CAD build for the part. Positions are in the model's coordinates, mm. Face numbers are marked on the shaded views. A direction names the side the tool comes from. Give positions to 0.01 mm unless a question says otherwise; leave off trailing zeros. Loops run counter-clockwise (first coordinate to the right, second up) from the corner with the lowest first, then second, coordinate; pieces in that order, holes last. Notation, with made-up numbers: (7.5, 55.25) - (27.5, 55.25) arc R16 ccw to (27.5, 64.25) - close; hole circle Ø8 at (85, 86.5). An arc over 180 degrees is marked (long way). Return JSON: item names as keys, results as strings.
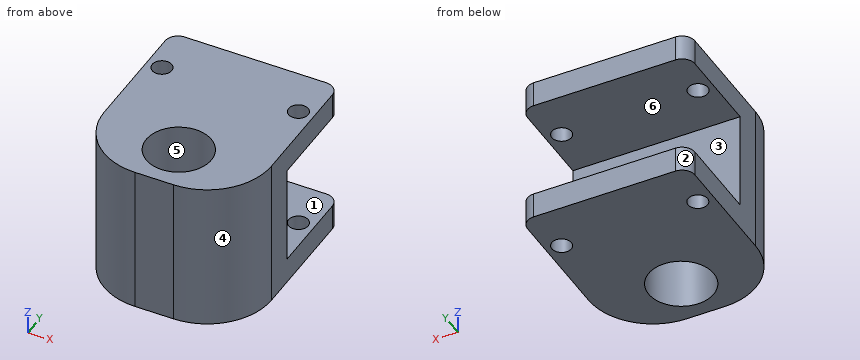
Autodesk Inventor part; units mm, degrees
ref_plane "YZ Plane" through (0, 0, 0) normal (1, 0, 0) x (0, 1, 0)
ref_plane "XZ Plane" through (0, 0, 0) normal (0, 1, 0) x (-1, 0, 0)
ref_plane "XY Plane" through (0, 0, 0) normal (0, 0, 1) x (1, 0, 0)
ref_plane "Work Plane1" through (0, 0, 0) normal (0, 0, 1) x (1, 0, 0)
sketch "Sketch1" plane through (0, 0, 0) normal (0, 0, 1) x (1, 0, 0)
  line L0 (-9.7566, -4.627) -> (-9.7566, 4.627) construction
  line L1 (-9.7566, -9.525) -> (-314.5566, -9.525) construction
  line L2 (-9.7566, 9.525) -> (-314.5566, 9.525) construction
  line L3 (-42.7766, 3) -> (-42.7766, -3) construction
  line L4 (-9.7566, 9.525) -> (-42.7766, 9.525)
  line L5 (-42.7766, 9.525) -> (-42.7766, -9.525)
  line L6 (-9.7566, -9.525) -> (-9.7566, 9.525)
  line L7 (-9.7566, -9.525) -> (-9.7566, -28.575)
  line L8 (-9.7566, -28.575) -> (-42.7766, -28.575)
  line L9 (-42.7766, -28.575) -> (-42.7766, -9.525)
  arc A0 (-38.0982, 0.6213) -> (-38.1469, -0.737) centre (-39.737, 0) ccw construction
  arc A1 (-11.1575, 0.6213) -> (-11.2061, -0.737) centre (-12.7962, 0) ccw construction
  circle A2 centre (-12.7962, 0) radius 1.9304
  circle A3 centre (-39.737, 0) radius 1.9304
  point P0 (0, 0)
  dimension "d1" = 19.05
  dimension "d2" = 3.8608
  dimension "d3" = 3.8608
extrude "Extrusion1" add sketch "Sketch1" along normal blind 5.08
ref_plane "Work Plane2" through (0, 0, -19.558) normal (0, 0, -1) x (-1, 0, 0)
sketch "Sketch2" plane through (0, 0, -19.558) normal (0, 0, -1) x (-1, 0, 0)
  line L0 (9.7566, -28.575) -> (9.7566, 9.525)
  line L1 (42.7766, 9.525) -> (42.7766, -28.575)
  line L2 (9.7566, 9.525) -> (42.7766, 9.525)
  line L3 (42.7766, 9.525) -> (42.7766, -28.575)
  line L4 (42.7766, -28.575) -> (9.7566, -28.575)
  line L5 (9.7566, -28.575) -> (9.7566, 9.525)
  circle A0 centre (12.7962, 0) radius 1.9304
  circle A1 centre (12.7962, 0) radius 1.9304
  circle A2 centre (39.6875, 0) radius 1.9304
  point P0 (0, 0)
  dimension "d7" = 3.8608
  dimension "d8" = 3.8608
  dimension "d24" = 38.1
  dimension "d25" = 9.525
  dimension "d26" = 26.8913
extrude "Extrusion2" add sketch "Sketch2" along normal blind 5.08
sketch "Sketch3" plane through (0, 0, 0) normal (0, 0, -1) x (-1, 0, 0)
  line L0 (9.7566, 9.525) -> (42.7766, 9.525) construction
  line L1 (9.7566, 9.525) -> (42.7766, 9.525) construction
  line L2 (42.7766, 9.525) -> (42.7766, -9.525) construction
  line L3 (42.7766, -9.525) -> (9.7566, -9.525) construction
  line L4 (9.7566, -9.525) -> (9.7566, 9.525) construction
  line L5 (42.7766, -28.575) -> (9.7566, -28.575)
  line L6 (42.7766, -10.033) -> (42.7766, -28.575)
  line L7 (42.7766, -28.575) -> (9.7566, -28.575)
  line L8 (9.7566, -28.575) -> (9.7566, -10.033)
  line L9 (42.7766, 9.525) -> (42.7766, -28.575)
  line L10 (42.7766, -10.033) -> (9.7566, -10.033)
  point P0 (0, 0)
  dimension "d11" = 19.05
extrude "Extrusion3" add sketch "Sketch3" along normal up to surface (19.558 mm away)
sketch "Sketch4" plane through (0, 0, -24.638) normal (0, 0, -1) x (-1, 0, 0)
  circle A0 centre (26.2666, -19.304) radius 6.4135
  line L0 (9.7566, -28.575) -> (42.7766, -28.575)
  line L1 (42.7766, -28.575) -> (42.7766, 9.525)
  line L2 (9.7566, 9.525) -> (9.7566, -28.575)
  line L3 (42.7766, -10.033) -> (9.7566, -10.033) construction
  point P0 (0, 0)
  dimension "d15" = 12.827
  dimension "d16" = 9.271
  dimension "d17" = 33.02
  dimension "d18" = 16.51
  dimension "d19" = 18.542
extrude "Extrusion4" cut sketch "Sketch4" against normal through all
fillet "Fillet1" radius 12.7 2 edges at (-9.7566, -28.575, -9.779) (-42.7766, -28.575, -9.779)
fillet "Fillet2" radius 2.54 4 edges at (-9.7566, 9.525, -22.098) (-9.7566, 9.525, 2.54) (-42.7766, 9.525, -22.098) (-42.7766, 9.525, 2.54)
equation "\"d16\" = 0.5 * d19"
equation "\"d18\" = 0.5 * d17"
properties part number "Bearing mount for xrail"
1. Pull direction Y, two halves, no side cores. Call the marked faces 3, 4, 5 and 6: +Y half, -Y half, draft (parallel to the pull), parting line (faces both ways), or undercut.
Values follow:
{"face 3": "+Y half", "face 4": "-Y half", "face 5": "undercut", "face 6": "draft"}
2. Cut at C-C, the plane z = -2.25. Write the cut outline in (x, y) (1 decimal), plus the area to 3 significant figures.
Values follow:
{"outline": "(-42.8, -15.9) arc R12.7 ccw to (-30.1, -28.6) - (-22.5, -28.6) arc R12.7 ccw to (-9.8, -15.9) - (-9.8, -10) - (-42.8, -10) - close; hole circle Ø12.8 at (-26.3, -19.3)", "area": "414 mm²"}
3. Which spindle directions (+Z, -Z, +X, -X, +Y, -Y) get a long thin tool onto all of the face, cutting with end or side? Do the marked faces 1 and 2. Say none if no direction does.
Values follow:
{"face 1": "+X, -X, +Y", "face 2": "+Z, -Z, -X, +Y"}
4. Drill centre lines: probe 1 along Z at (x, y) = (-26.5, -10); probe 2 along Y at (x, z) = (-30.5, -7.75); probe 3 along Y at (x, z) = (-28.5, -3.25) (3 decimals). Where is each one in solid material? Low to high.
Values follow:
{"probe 1": "z = -24.64 to -19.56, 0 to 5.08", "probe 2": "y = -28.57 to -24.12, -14.49 to -10.03", "probe 3": "y = -28.575 to -25.316, -13.292 to -10.033"}
5. Cut at D-D, the plane y = -21. Write the cut outline in (x, z), plus the area to 3 significant figures.
Values follow:
{"outline": "(-41.7, -24.64) - (-32.45, -24.64) - (-32.45, 5.08) - (-41.7, 5.08) - close; (-20.08, -24.64) - (-10.84, -24.64) - (-10.84, 5.08) - (-20.08, 5.08) - close", "area": "549 mm²"}
6. Cut at A-A, the plane y = 0. Write the cut outline in (x, z).
Values follow:
{"outline": "(-42.78, -24.64) - (-41.62, -24.64) - (-41.62, -19.56) - (-42.78, -19.56) - close; (-42.78, 0) - (-41.67, 0) - (-41.67, 5.08) - (-42.78, 5.08) - close; (-37.81, 0) - (-14.73, 0) - (-14.73, 5.08) - (-37.81, 5.08) - close; (-37.76, -24.64) - (-14.73, -24.64) - (-14.73, -19.56) - (-37.76, -19.56) - close; (-10.87, -24.64) - (-9.76, -24.64) - (-9.76, -19.56) - (-10.87, -19.56) - close; (-10.87, 0) - (-9.76, 0) - (-9.76, 5.08) - (-10.87, 5.08) - close"}
7. Cut at B-B, the plane x = -14. Write the cut outline in (y, z) (3 decimals), plus the area to 3 significant figures.
Values follow:
{"outline": "(-25.35, -24.638) - (-1.509, -24.638) - (-1.509, -19.558) - (-10.033, -19.558) - (-10.033, 0) - (-1.509, 0) - (-1.509, 5.08) - (-25.35, 5.08) - close; (1.509, -24.638) - (9.525, -24.638) - (9.525, -19.558) - (1.509, -19.558) - close; (1.509, 0) - (9.525, 0) - (9.525, 5.08) - (1.509, 5.08) - close", "area": "623 mm²"}
8. Drop a flat-ended pin along its axis: P1, Ø6, axis at x = -22.5, z = -5.5, coming from the +Y side. Give the stop position or say it passes through.
Values follow:
{"P1": "stops at y = -10.03"}
